```python
from build123d import *

# Parameters (mm, degrees)
F1_DEPTH = 30
F2_DEPTH = 20
F3_W     = 61.814844
F3_H     = 59.7312
F4_DEPTH = 50
F6_DEPTH = 60


with BuildPart() as f1:
    # F0 (on Right) → F1 (new body)
    with BuildSketch(Plane.YZ):
        with BuildLine():
            ThreePointArc((50, -145), (44.72136, -122.63932), (30, -105))
            ThreePointArc((30, -105), (0, -95), (-30, -105))
            ThreePointArc((-30, -105), (-22.36068, -189.72136), (50, -145))
        make_face()
    extrude(amount=F1_DEPTH)

    # F0 (on Right) → F2 (join)
    with BuildSketch(Plane.YZ):
        with BuildLine():
            Line((30, -105), (30, 145))
            Line((30, 145), (-30, 145))
            Line((-30, 145), (-30, -105))
            ThreePointArc((-30, -105), (0, -95), (30, -105))
        make_face()
        with BuildLine():
            ThreePointArc((50, -145), (44.72136, -122.63932), (30, -105))
            ThreePointArc((30, -105), (0, -95), (-30, -105))
            ThreePointArc((-30, -105), (-22.36068, -189.72136), (50, -145))
        make_face()
    extrude(amount=F2_DEPTH)

    # F3 (on Front) → F4 (cut, symmetric)
    with BuildSketch(Plane.XZ):
        with Locations((-90.155922, 117.482759)):
            Rectangle(F3_W, F3_H)
    extrude(amount=F4_DEPTH, both=True, mode=Mode.SUBTRACT)

    # F5 (on face) → F6 (join)
    with BuildSketch(Plane(origin=(0, 30, 0), x_dir=(-1, 0, 0), z_dir=(0, 1, 0))):
        with BuildLine():
            ThreePointArc((0, 145), (68.472419, 192.411567), (150, 209.428685))
            Line((150, 209.428685), (150, 229.428685))
            ThreePointArc((150, 229.428685), (54.480666, 208.395375), (-20, 145))
            Line((-20, 145), (0, 145))
        make_face()
    extrude(amount=-F6_DEPTH)

    # F7: F1 across face


with BuildPart() as f1_1:
    add(f1.part)
    add(f1.part.mirror(Plane(origin=(-150, 0, 219.428685), x_dir=(0, -1, 0), z_dir=(-1, 0, 0))))


solid = f1_1.part
```
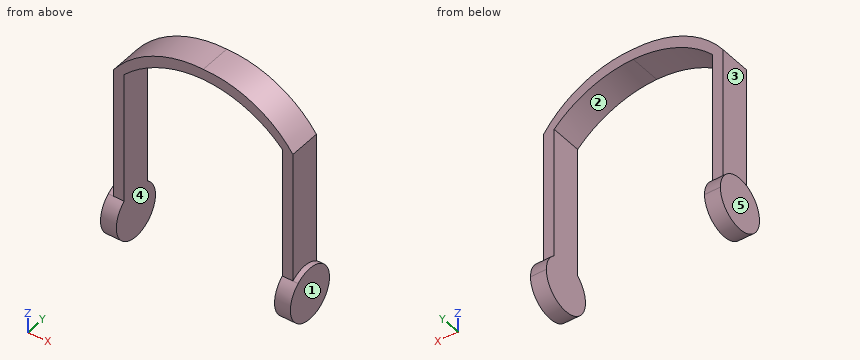
Work out the finished part from the listing and answer in its coordinate system (mm). Face numbers are marked on the shaded views. A direction names the side the tool comes from. Round coordinates to 2 decimals unless told otherwise and drop trailing zeros. Write each loop counter-clockwise with the first axis right and the second up, starting at its lowest first coordinate (ties: lowest second). Pieces come first, ordered by that corner, then holes. Notation, with made-up numbers: (-39, 51) - (-22, 51) arc R16 cw to (-22, 66) - close; hole circle Ø3 at (43.25, 41). An arc over 180 degrees is marked (long way). Return JSON: item names as keys, results as strings. Group by question number.
Q1. The mould has two halves that part along X. Classify the marked faces 1, 2 and 3: released by +X, released by -X, zero draft, split by the parting line, or undercut.
Q2. The part is cut by section D-D on x = -42. Write down the section's boundary in (y, z).
Q3. The part is cut by section C-C on y = 18.5. Write down the section's boundary in (x, z).
Q4. The part is cut by section A-A on y = 40. Write down the section's boundary in (x, z), then the cut area to 3 significant figures.
Q5. For the marked faces 4 and 5, determine the directions among +Z, -Z, +X, -X, +Y, -Y from which every point of the face is accessible in a straight line to the end or side of a thin tool.
Q6. Find the intervals of material crossed by L1, parallel to X at y = 8.5, z = 35.5; L2, parallel to Y at x = -313, z = -18; L3, parallel to Z at x = -148, y = -25, in increasing order.
Q7. The part is cut by section B-B on z = 68. Write down the section's boundary in (x, y), then the cut area to 3 significant figures.
Q8. Each of these flat-tipped pins is pushed along its axis until it touches: pin 1 Ø10 at (x, y) = (-84.5, -22.5) entering from -Z; pin 2 Ø12 at (x, y) = (-179, 39) entering from -Z; pin 3 Ø4 at (y, z) = (10, 14) entering from -X; pin 4 Ø1 at (x, y) = (-174, 24) entering from +Z. Where does it stop, or does it pass through?
Solved:
{
 "1": {"face 1": "released by +X", "face 2": "undercut", "face 3": "released by -X"},
 "2": {"outline": "(-30, 178.74) - (30, 178.74) - (30, 201.64) - (-30, 201.64) - close"},
 "3": {"outline": "(-330, -191.45) - (-300, -191.45) - (-300, 145) arc R209.69 cw to (-150, 209.43) arc R209.69 cw to (0, 145) - (0, -191.45) - (30, -191.45) - (30, -98.55) - (20, -98.55) - (20, 145) arc R202.25 ccw to (-150, 229.43) arc R202.25 ccw to (-320, 145) - (-320, -98.55) - (-330, -98.55) - close"},
 "4": {"outline": "(-330, -175) - (-300, -175) - (-300, -115) - (-330, -115) - close; (0, -175) - (30, -175) - (30, -115) - (0, -115) - close", "area": "3,600 mm²"},
 "5": {"face 4": "-Z, +Y, -Y", "face 5": "+Z, -Z, -X, +Y, -Y"},
 "6": {"L1": "-320 to -300, 0 to 20", "L2": "-30 to 30", "L3": "209.41 to 229.47"},
 "7": {"outline": "(-320, -30) - (-300, -30) - (-300, 30) - (-320, 30) - close; (0, -30) - (20, -30) - (20, 30) - (0, 30) - close", "area": "2,400 mm²"},
 "8": {"pin 1": "z = 196.78", "pin 2": "through", "pin 3": "x = -320", "pin 4": "z = 228.71"}
}
